Read the model definition and answer for the solid it produces. Units are mm, in the model's axes. Round coordinates to 2 decimals unless told otherwise and drop trailing zeros. Order: outer loops, then holes, each group sorted by start corner. A loop starts at its lowest first (then second) coordinate and runs counter-clockwise, first axis right, second up.
from build123d import *

# Parameters (mm, degrees)
F0_W     = 90
F0_H     = 3.175
F1_DEPTH = 70
F3_D     = 4.4


with BuildPart() as f1:
    # F0 (on Top) → F1 (new body)
    with BuildSketch(Plane.XY):
        Rectangle(F0_W, F0_H)
    extrude(amount=F1_DEPTH)

    # F3 (through all)
    with Locations(Plane(origin=(0, 1.5875, 0), x_dir=(-1, 0, 0), z_dir=(0, 1, 0))):
        with Locations((33.8875, 22.5), (33.8875, 47.5), (-3.175, 62.0625)):
            Hole(F3_D / 2)


solid = f1.part
Q1. For a pull along X with two mould halves and no side action, classify faces 1 (the face through (2.698, -0.022, 59.915)), 2 (the face through (-45, 0, 35)), 3 (the face through (-1, 0, 70)) as released by +X, released by -X, zero draft, split by the parting line, or undercut.
Outcome:
face 1: undercut
face 2: released by -X
face 3: zero draft
Q2. A cutting plane is placed at A-A, the plane z = 22.5. Give the vertices of the cut face in (x, y).
Outcome:
outline: (-45, -1.59) - (-36.09, -1.59) - (-36.09, 1.59) - (-45, 1.59) - close; (-31.69, -1.59) - (45, -1.59) - (45, 1.59) - (-31.69, 1.59) - close
Q3. Straight lines are drawn through the part: probe 1 along X at (y, z) = (1.15, 60.5); probe 2 along X at (y, z) = (-0.5, 24). For each, find the intervals that lie inside material, in ascending order.
Outcome:
probe 1: x = -45 to 1.63, 4.72 to 45
probe 2: x = -45 to -35.5, -32.28 to 45
Q4. A flat-ended cylindrical pin translates along its axis: pin 1 (7 mm diameter, centred on x = -33.89, z = 47.5, fed in from +Y). Find the tip coordinate at first contact, or state that the pin passes through.
Outcome:
pin 1: stops at y = 1.59
